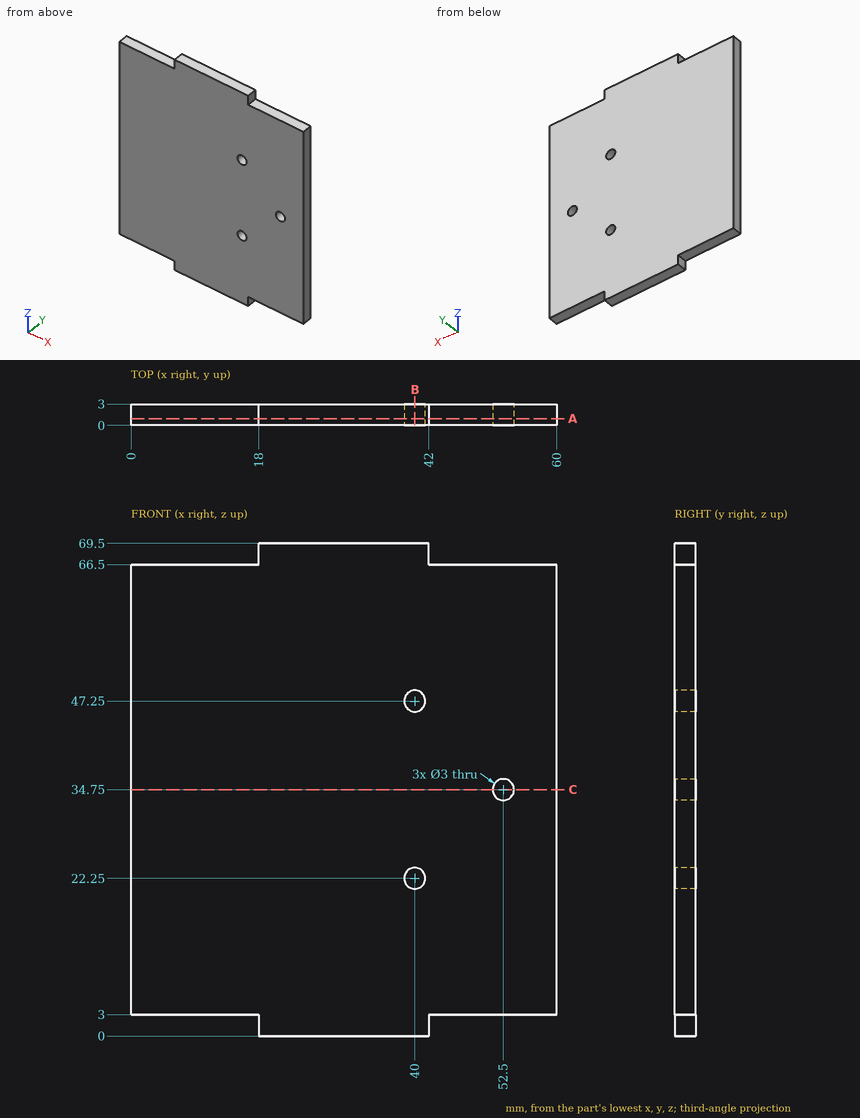
Verification items for this drawing (mm, ordinates from the low corner). Give positions to 0.01 mm unless a question says otherwise; leave off trailing zeros. Loops run counter-clockwise (first coordinate to the right, second up) from the corner with the lowest first, then second, coordinate; pieces in that order, holes last.
1. Cross-section at A-A on y = 0.95. Record the cut outline in (x, z), and give its area (3 significant figures).
Derived:
outline: (0, 3) - (18, 3) - (18, 0) - (42, 0) - (42, 3) - (60, 3) - (60, 66.5) - (42, 66.5) - (42, 69.5) - (18, 69.5) - (18, 66.5) - (0, 66.5) - close; hole circle Ø3 at (40, 22.25); hole circle Ø3 at (40, 47.25); hole circle Ø3 at (52.5, 34.75)
area: 3,930 mm2
2. Cross-section at B-B on x = 40. Record the cut outline in (y, z), and give its area (4 significant figures).
Derived:
outline: (0, 0) - (3, 0) - (3, 20.75) - (0, 20.75) - close; (0, 23.75) - (3, 23.75) - (3, 45.75) - (0, 45.75) - close; (0, 48.75) - (3, 48.75) - (3, 69.5) - (0, 69.5) - close
area: 190.5 mm2
3. Go/stop test with flat-tipped pins: P1, Ø1.5, axis at y = 1.5, z = 67.5, coming from the +X side; P2, Ø1, axis at x = 53.5, y = 2, coming from the +Z side; P3, Ø1.5, axis at y = 1.5, z = 68, coming from the -X side. Record where each tip stops, or that it passes through.
Derived:
P1: stops at x = 42
P2: stops at z = 66.5
P3: stops at x = 18
4. Cross-section at C-C on z = 34.75. Record the cut outline in (x, y).
Derived:
outline: (0, 0) - (51, 0) - (51, 3) - (0, 3) - close; (54, 0) - (60, 0) - (60, 3) - (54, 3) - close
5. Material ranges on probe 1 along Z at (x, y) = (40, 1); probe 2 along Z at (x, y) = (52.5, 0.95); probe 3 along Z at (x, y) = (42.5, 2.3), recorded low to high.
Derived:
probe 1: z = 0 to 20.75, 23.75 to 45.75, 48.75 to 69.5
probe 2: z = 3 to 33.25, 36.25 to 66.5
probe 3: z = 3 to 66.5
